Source: CAD feature listing. Evaluate the final solid. Frame: model axes, mm. A direction names the side the tool comes from. Round coordinates to 2 decimals unless told otherwise and drop trailing zeros. Order: outer loops, then holes, each group sorted by start corner. A loop starts at its lowest first (then second) coordinate and runs counter-clockwise, first axis right, second up. Notation, with made-up numbers: M 51.5,65.25 L 92.5,65.25 A19 cw 92.5,98.25 Z; hole C -9,60 d7. An arc over 180 degrees is marked long. Use one line per item in the form item = value. Start each with the question number.
Q1. Section A-A (y = 10). Return the cut outline in (x, z), plus the area to 3 significant figures.
Q2. Section C-C (x = 38.5). Return the cut outline in (y, z).
Q3. Material intervals for probe 1 along X at (y, z) = (13.25, -5.25); probe 2 along Z at (x, y) = (29, 4.25); probe 3 along Z at (x, y) = (43.5, 6.5), sorted ascending.
Q4. Section D-D (z = -2.5). Return the cut outline in (x, y).
Q5. Reachability of faces 1 (the cylindrical face through (45.857, 8.699, 9.062)), 2 (the flat face through (42, 10, 0)), 3 (the flat face through (40, 10, -2)) from +Z, -Z, +X, -X, +Y, -Y: full face, straight path, thin tool, end or side. Return the list, or none.
Q6. Section B-B (z = 8). Return the cut outline in (x, y).
Q7. Contact query for flat-ended pins moving along their axis: pin 1 (6 mm diameter, centred on x = 23.5, y = 9.5, fed in from +Z); pin 2 (5 mm diameter, centred on y = 7, z = 4.5, fed in from -X); pin 3 (6.5 mm diameter, centred on x = 44, y = 9.5, fed in from -Z); pin 4 (3 mm diameter, centred on y = 9.5, z = -4.5, fed in from +X). Output: stop coordinate, or through.
from build123d import *

# Parameters (mm, degrees)
SKETCH1_W           = 40
SKETCH1_H           = 20
BOSS_EXTRUDE1_DEPTH = 10
SKETCH2_R           = 6
BOSS_EXTRUDE2_DEPTH = 15


with BuildPart() as part:
    # Sketch1 → Boss-Extrude1 (new, symmetric)
    with BuildSketch(Plane.XY):
        with Locations((20, 10)):
            Rectangle(SKETCH1_W, SKETCH1_H)
    extrude(amount=BOSS_EXTRUDE1_DEPTH, both=True)

    # Sketch2 → Boss-Extrude2 (add)
    with BuildSketch(Plane.XY):
        with Locations(Location((40, 10, 0), (0, 0, 90))):
            Circle(SKETCH2_R)
    extrude(amount=BOSS_EXTRUDE2_DEPTH)


solid = part.part
Results list:
q1.outline = M 0,-10 L 40,-10 L 40,0 L 46,0 L 46,15 L 34,15 L 34,10 L 0,10 Z
q1.area = 920 mm2
q2.outline = M 0,-10 L 20,-10 L 20,10 L 15.81,10 L 15.81,15 L 4.19,15 L 4.19,10 L 0,10 Z
q3.probe_1 = 0 to 40
q3.probe_2 = -10 to 10
q3.probe_3 = 0 to 15
q4.outline = M 0,0 L 40,0 L 40,20 L 0,20 Z
q5.face_1 = +Z
q5.face_2 = -Z, +X, +Y, -Y
q5.face_3 = -Z, +X
q6.outline = M 0,0 L 40,0 L 40,4 A6 ccw 40,16 L 40,20 L 0,20 Z
q7.pin_1 = 10
q7.pin_2 = 0
q7.pin_3 = 0
q7.pin_4 = 40
